Read the model definition and answer for the solid it produces. Units are mm, in the model's axes. Face numbers are marked on the shaded views. A direction names the side the tool comes from. Round coordinates to 2 decimals unless told otherwise and drop trailing zeros. Order: outer loops, then holes, each group sorted by start corner. A loop starts at its lowest first (then second) coordinate and runs counter-clockwise, first axis right, second up. Notation, with made-up numbers: (18.5, 67.5) - (66.5, 67.5) arc R16 cw to (66.5, 74.5) - close; hole circle Ø2 at (48.25, 13). An arc over 180 degrees is marked (long way). Answer as a JSON object with one key per item and string values. Group by question number.
Q1. The mould has two halves that part along Z. Classify the marked faces 1, 2 and 3: pulls with the +Z half, pulls with the -Z half, needs draft (parallel to the pull), parting line crosses it, or undercut.
Q2. A tool of negligible diameter and unlimited length cuts with its end or side. For the marked faces 4 and 5, from which of +Z, -Z, +X, -X, +Y, -Y can it reach the whole face along a straight path? Write none if from no direction.
Q3. A cutting plane is placed at B-B on x = 202. Determine the outline of the cut face in (y, z).
Q4. A cutting plane is placed at A-A on y = -38.1. Determine the outline of the cut face in (x, z) (1 decimal).
Q5. Consider line 1 (Z direction, x = 213.5, y = -71.5); line 2 (X direction, y = -34, z = 24.5) (3 decimals); line 3 (X direction, y = -36, z = 50) (3 decimals). Determine where each line is inside the solid, lowest interval first.
Q6. Given pin 1 Ø3 at (x, y) = (48, -12.5) entering from +Z; pin 2 Ø10 at (x, y) = (187.325, -38.1) entering from +Z, each flat-ended and moving along its own axis, determine where each tip first touches the part or whether it passes through.
Q7. A cutting plane is placed at C-C on y = -23. Determine the outline of the cut face in (x, z) (1 decimal).
Q8. A cutting plane is placed at D-D on z = 79.5. Determine the outline of the cut face in (x, y) (1 decimal), and give its area (3 significant figures).
```python
from build123d import *

# Parameters (mm, degrees)
F0_R     = 11.1125
F1_DEPTH = 76.2
F2_R     = 6.35
F3_DEPTH = 81.026
F4_R     = 7.9375
F5_DEPTH = 65.278


with BuildPart() as f1:
    # F0 (on Front) → F1 (new body)
    with BuildSketch(Plane.XZ):
        with BuildLine():
            Line((225.425, 152.4), (76.2, 152.4))
            ThreePointArc((76.2, 152.4), (22.318463, 130.081537), (0, 76.2))
            ThreePointArc((0, 76.2), (22.318463, 22.318463), (76.2, 0))
            Line((76.2, 0), (225.425, 0))
            Line((225.425, 0), (225.425, 50.8))
            Line((225.425, 50.8), (149.225, 50.8))
            Line((149.225, 50.8), (149.225, 101.6))
            Line((149.225, 101.6), (225.425, 101.6))
            Line((225.425, 101.6), (225.425, 152.4))
        make_face()
        with Locations((111.125, 76.2)):
            Circle(F0_R, mode=Mode.SUBTRACT)
    extrude(amount=F1_DEPTH)

    # F2 (on face) → F3 (cut)
    with BuildSketch(Plane.XY.offset(152.4)):
        with Locations((187.325, -38.1)):
            Circle(F2_R)
    extrude(amount=-F3_DEPTH, mode=Mode.SUBTRACT)

    # F4 (on face) → F5 (cut)
    with BuildSketch(Plane.XY.offset(50.8)):
        with Locations((187.325, -38.1)):
            Circle(F4_R)
    extrude(amount=-F5_DEPTH, mode=Mode.SUBTRACT)


solid = f1.part
```
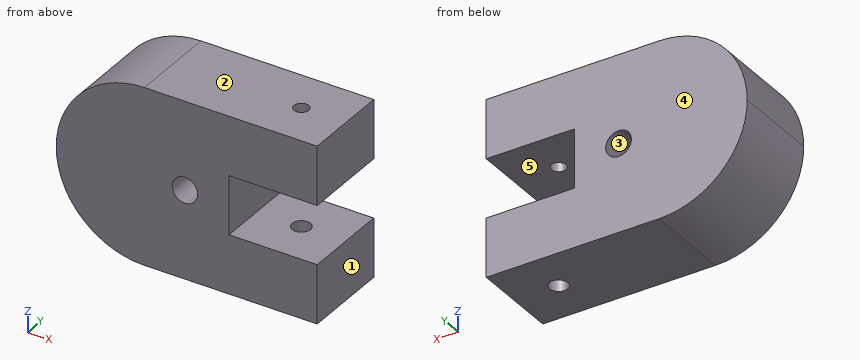
Result set:
{
 "1": {"face 1": "needs draft", "face 2": "pulls with the +Z half", "face 3": "undercut"},
 "2": {"face 4": "+Z, -Z, +X, -X, +Y", "face 5": "+X, +Y, -Y"},
 "3": {"outline": "(-76.2, 0) - (0, 0) - (0, 50.8) - (-76.2, 50.8) - close; (-76.2, 101.6) - (0, 101.6) - (0, 152.4) - (-76.2, 152.4) - close"},
 "4": {"outline": "(0, 76.2) arc R76.2 ccw to (76.2, 0) - (179.4, 0) - (179.4, 50.8) - (149.2, 50.8) - (149.2, 101.6) - (181, 101.6) - (181, 152.4) - (76.2, 152.4) arc R76.2 ccw to start; (193.7, 101.6) - (225.4, 101.6) - (225.4, 152.4) - (193.7, 152.4) - close; (195.3, 0) - (225.4, 0) - (225.4, 50.8) - (195.3, 50.8) - close; hole circle Ø22.2 at (111.1, 76.2)"},
 "5": {"line 1": "z = 0 to 50.8, 101.6 to 152.4", "line 2": "x = 20.222 to 180.528, 194.122 to 225.425", "line 3": "x = 4.646 to 179.67, 194.98 to 225.425"},
 "6": {"pin 1": "stops at z = 147.57", "pin 2": "passes through"},
 "7": {"outline": "(0, 76.2) arc R76.2 ccw to (76.2, 0) - (225.4, 0) - (225.4, 50.8) - (149.2, 50.8) - (149.2, 101.6) - (225.4, 101.6) - (225.4, 152.4) - (76.2, 152.4) arc R76.2 ccw to start; hole circle Ø22.2 at (111.1, 76.2)"},
 "8": {"outline": "(0.1, -76.2) - (100.5, -76.2) - (100.5, 0) - (0.1, 0) - close; (121.7, -76.2) - (149.2, -76.2) - (149.2, 0) - (121.7, 0) - close", "area": "9,750 mm²"}
}
